from build123d import *

# Parameters (mm, degrees)
SKETCH1_R                  = 3.75
BOSS_EXTRUDE1_DEPTH        = 10.5
F_3_5_3_5_DIAMETER_HOLE1_D = 3.5
SKETCH5_R                  = 4.75
SKETCH5_R_2                = 3.75
BOSS_EXTRUDE2_DEPTH        = 3.5


with BuildPart() as part:
    # Sketch1 → Boss-Extrude1 (new body)
    with BuildSketch(Plane(origin=(0, 0, 0), x_dir=(1, 0, 0), z_dir=(0, 1, 0))):
        with Locations(Location((0, 0, 0), (0, 0, 90))):
            Circle(SKETCH1_R)
    extrude(amount=BOSS_EXTRUDE1_DEPTH)

    # Ø3.5 (3.5) Diameter Hole1 (through all)
    with Locations(Plane(origin=(0, 10.5, 0), x_dir=(1, 0, 0), z_dir=(0, 1, 0))):
        with Locations((0, 0)):
            Hole(F_3_5_3_5_DIAMETER_HOLE1_D / 2)

    # Sketch5 → Boss-Extrude2 (add)
    with BuildSketch(Plane.XZ):
        with Locations(Location((0, 0, 0), (0, 0, 270))):
            Circle(SKETCH5_R)
        with Locations(Location((0, 0, 0), (0, 0, 270))):
            Circle(SKETCH5_R_2, mode=Mode.SUBTRACT)
    extrude(amount=-BOSS_EXTRUDE2_DEPTH)


solid = part.part
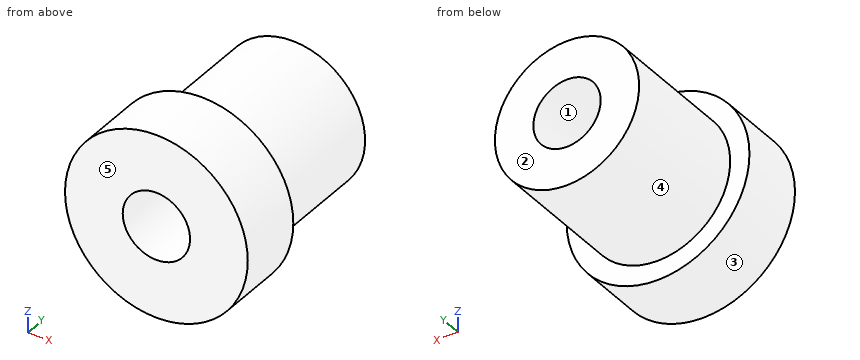
Model file for the job. Use its own axes, mm. Face numbers are marked on the shaded views. A direction names the side the tool comes from. Coordinates: 2 decimals unless noted, no trailing zeros. Write each loop counter-clockwise with the first axis right and the second up, starting at its lowest first coordinate (ties: lowest second). Pieces come first, ordered by that corner, then holes. Notation, with made-up numbers: (7.25, 82) -> (40.25, 82) arc R17 cw to (40.25, 102) -> close; hole circle Ø4 at (64.25, 52). An arc over 180 degrees is marked (long way). One line per item, written item: value. Start each with the question number.
1) Slice it at D-D on z = -2.5. Write the cut outline in (x, y), then the cut area to 3 significant figures.
2) Slice it at B-B on z = 0. Write the cut outline in (x, y), then the cut area to 3 significant figures.
3) Slice it at C-C on y = 1.5. Write the cut outline in (x, z), then the cut area to 3 significant figures.
4) Flat gauge pin, fed straight in: pin 1 Ø4 at (x, y) = (-3, 8) entering from -Z. Where does the tip first touch, or does it go through?
5) Slice it at A-A on x = 0. Write the cut outline in (y, z).
6) Pull direction X, two halves, no side cores. Call the marked faces 1, 2 and 3: +X half, -X half, draft (parallel to the pull), parting line (faces both ways), or undercut.
7) Probe probe 1 along Z at (x, y) = (0, 6.5); probe 2 along X at (y, z) = (5.25, 1.5); probe 3 along Z at (x, y) = (0.75, 2). List the from-to ranges inside material, lowest first.
8) Which spindle directions (+Z, -Z, +X, -X, +Y, -Y) get a long thin tool onto all of the face, cutting with end or side? Do the marked faces 4 and 5. Say none if no direction does.
Answers follow:
1. outline: (-4.04, 0) -> (4.04, 0) -> (4.04, 3.5) -> (2.8, 3.5) -> (2.8, 10.5) -> (-2.8, 10.5) -> (-2.8, 3.5) -> (-4.04, 3.5) -> close
1. area: 67.4 mm2
2. outline: (-4.75, 0) -> (-1.75, 0) -> (-1.75, 10.5) -> (-3.75, 10.5) -> (-3.75, 3.5) -> (-4.75, 3.5) -> close; (1.75, 0) -> (4.75, 0) -> (4.75, 3.5) -> (3.75, 3.5) -> (3.75, 10.5) -> (1.75, 10.5) -> close
2. area: 49.0 mm2
3. outline: circle Ø9.5 at (0, 0); hole circle Ø3.5 at (0, 0)
3. area: 61.3 mm2
4. pin 1: z = -3.61
5. outline: (0, -4.75) -> (3.5, -4.75) -> (3.5, -3.75) -> (10.5, -3.75) -> (10.5, -1.75) -> (0, -1.75) -> close; (0, 1.75) -> (10.5, 1.75) -> (10.5, 3.75) -> (3.5, 3.75) -> (3.5, 4.75) -> (0, 4.75) -> close
6. face 1: undercut
6. face 2: draft
6. face 3: parting line
7. probe 1: -3.75 to -1.75, 1.75 to 3.75
7. probe 2: -3.44 to -0.9, 0.9 to 3.44
7. probe 3: -4.69 to -1.58, 1.58 to 4.69
8. face 4: +Y
8. face 5: +Z, -Z, +X, -X, -Y
